```python
from build123d import *

# Parameters (mm, degrees)
F0_R     = 203.2
F1_DEPTH = 1016
F2_W     = 127
F2_H     = 457.2
F3_DEPTH = 812.801
F2_W_2   = 635
F2_W_3   = 279.4
F4_DEPTH = 812.801
F5_W     = 812.8
F5_H     = 279.4
F6_DEPTH = 635.001
F8_DEPTH = 812.8


with BuildPart() as f1:
    # F0 (on Front) → F1 (new body)
    with BuildSketch(Plane.XZ):
        with BuildLine():
            ThreePointArc((0, -406.4), (287.368196, -287.368196), (406.4, 0))
            ThreePointArc((406.4, 0), (287.368196, 287.368196), (0, 406.4))
            ThreePointArc((0, 406.4), (-406.4, 0), (0, -406.4))
        make_face()
        Circle(F0_R, mode=Mode.SUBTRACT)
        with BuildLine():
            ThreePointArc((0, 406.4), (287.368196, 287.368196), (406.4, 0))
            ThreePointArc((406.4, 0), (287.368196, -287.368196), (0, -406.4))
            Line((0, -406.4), (914.4, -406.4))
            Line((914.4, -406.4), (914.4, -228.6))
            Line((914.4, -228.6), (1727.2, -228.6))
            Line((1727.2, -228.6), (1727.2, 228.6))
            Line((1727.2, 228.6), (914.4, 228.6))
            Line((914.4, 228.6), (914.4, 406.4))
            Line((914.4, 406.4), (0, 406.4))
        make_face()
    extrude(amount=F1_DEPTH)

    # F2 (on face) → F3 (cut, through all)
    with BuildSketch(Plane.XY.offset(406.4)):
        with Locations((-342.9, -508)):
            Rectangle(F2_W, F2_H)
    extrude(amount=-F3_DEPTH, mode=Mode.SUBTRACT)

    # F2 (on face) → F4 (cut, through all)
    with BuildSketch(Plane.XY.offset(406.4)):
        with Locations((317.5, -508)):
            Rectangle(F2_W_2, F2_H)
        with Locations((-139.7, -508)):
            Rectangle(F2_W_3, F2_H)
        with Locations((-342.9, -508)):
            Rectangle(F2_W, F2_H)
    extrude(amount=-F4_DEPTH, mode=Mode.SUBTRACT)

    # F5 (on face) → F6 (cut, through all)
    with BuildSketch(Plane.XY.offset(228.6)):
        with Locations((1320.8, -139.7)):
            Rectangle(F5_W, F5_H)
        with Locations((1320.8, -876.3)):
            Rectangle(F5_W, F5_H)
    extrude(amount=-F6_DEPTH, mode=Mode.SUBTRACT)

    # F7 (on face) → F8 (cut)
    with BuildSketch(Plane.YZ.offset(1727.2)):
        with BuildLine():
            ThreePointArc((-508, 228.6), (-346.35539, 161.64461), (-279.4, 0))
            Line((-279.4, 0), (-279.4, 228.6))
            Line((-279.4, 228.6), (-508, 228.6))
        make_face()
        with BuildLine():
            Line((-279.4, -228.6), (-279.4, 0))
            ThreePointArc((-279.4, 0), (-346.35539, -161.64461), (-508, -228.6))
            Line((-508, -228.6), (-279.4, -228.6))
        make_face()
        with BuildLine():
            Line((-736.6, -228.6), (-508, -228.6))
            ThreePointArc((-508, -228.6), (-669.64461, -161.64461), (-736.6, -1e-06))
            Line((-736.6, -1e-06), (-736.6, -228.6))
        make_face()
        with BuildLine():
            ThreePointArc((-736.6, -1e-06), (-669.64461, 161.64461), (-508, 228.6))
            Line((-508, 228.6), (-736.6, 228.6))
            Line((-736.6, 228.6), (-736.6, -1e-06))
        make_face()
    extrude(amount=-F8_DEPTH, mode=Mode.SUBTRACT)


solid = f1.part
```
Can you work these out from the model? Positions are in its coordinate system, mm. A direction names the side the tool comes from. Round coordinates to 2 decimals unless told otherwise and drop trailing zeros. Loops run counter-clockwise (first coordinate to the right, second up) from the corner with the lowest first, then second, coordinate; pieces in that order, holes last. Notation, with made-up numbers: M 62,82.5 L 74,82.5 A34 cw 74,115.5 Z; hole C 68,18 d2. An arc over 180 degrees is marked long. Answer in a Markdown table with one row per item.
1. Please list where these lines run through material, in increasing order: line 1 (Y direction, x = 356, z = -197.5); line 2 (Z direction, x = 0, y = -813.5); line 3 (X direction, y = -949, z = 0). Write a range as from..to.
Established:
| item | result |
|---|---|
| line 1 | -1016..-736.6, -279.4..0 |
| line 2 | -406.4..-203.2, 203.2..406.4 |
| line 3 | -406.4..-203.2, 203.2..914.4 |
2. If we section it at A-A, the plane x = -92.5: Please give me the cut outline in (y, z), plus the area to 3 significant figures.
Established:
| item | result |
|---|---|
| outline | M -1016,-395.73 L -736.6,-395.73 L -736.6,-180.93 L -1016,-180.93 Z; M -1016,180.93 L -736.6,180.93 L -736.6,395.73 L -1016,395.73 Z; M -279.4,-395.73 L 0,-395.73 L 0,-180.93 L -279.4,-180.93 Z; M -279.4,180.93 L 0,180.93 L 0,395.73 L -279.4,395.73 Z |
| area | 240,000 mm² |
3. On a 3-axis mill with a long thin cutter (end or side, diameter ignored), from which of +Z, -Z, +X, -X, +Y, -Y can I reach the whole of each face in a straight line? I mean faces 5 (the face through (914.4, -275, -6)), 6 (the face through (223, -736.6, 6)), 7 (the face through (392, 0, 6)). Say none if no direction works.
Established:
| item | result |
|---|---|
| face 5 | +X |
| face 6 | +Z, -Z, -X |
| face 7 | +Z, -Z, +X, -X, +Y |
4. If we section it at C-C, the plane z = -259.5: Please give me the cut outline in (x, y).
Established:
| item | result |
|---|---|
| outline | M -312.76,-1016 L 914.4,-1016 L 914.4,0 L -312.76,0 L -312.76,-279.4 L 635,-279.4 L 635,-736.6 L -312.76,-736.6 Z |
5. If we section it at D-D, the plane x = 1445: Please give me the cut outline in (y, z).
Established:
| item | result |
|---|---|
| outline | M -736.6,0 A228.6 ccw -508,-228.6 A228.6 ccw -279.4,0 A228.6 ccw -508,228.6 A228.6 ccw Z |
6. If we section it at B-B, the plane y = -539: Please give me the cut outline in (x, z), plus the area to 3 significant figures.
Established:
| item | result |
|---|---|
| outline | M 635,-406.4 L 914.4,-406.4 L 914.4,-226.49 L 1727.2,-226.49 L 1727.2,226.49 L 914.4,226.49 L 914.4,406.4 L 635,406.4 Z |
| area | 595,000 mm² |
7. I'm going to push flat-ended pins straight in: pin 1 Ø1.5 at (x, y) = (946.5, -488.5) entering from +Z; pin 2 Ø12 at (y, z) = (-495.5, -129) entering from -X; pin 3 Ø3 at (x, y) = (1489.5, -329) entering from +Z. Where does each tip first touch, or does it pass through?
Established:
| item | result |
|---|---|
| pin 1 | z = 227.83 |
| pin 2 | x = 635 |
| pin 3 | z = 144.05 |
8. Thinking about a two-plate mould opening in Z: for faces 1 (the face through (1727.2, -505, -3)), 2 (the face through (667, -501, 406.4)), 3 (the face through (-44.05, -874.344, -198.368)), 4 (the face through (-44.05, -137.744, -198.368)), which applies, pulls with the +Z half, pulls with the -Z half, needs draft (parallel to the pull), parting line crosses it, or undercut?
Established:
| item | result |
|---|---|
| face 1 | needs draft |
| face 2 | pulls with the +Z half |
| face 3 | undercut |
| face 4 | undercut |
